Design review of the part built by this model. Coordinates are the model's own, in mm. Give positions to 0.01 mm unless a question says otherwise; leave off trailing zeros. Order: outer loops, then holes, each group sorted by start corner. A loop starts at its lowest first (then second) coordinate and runs counter-clockwise, first axis right, second up. Notation, with made-up numbers: (42.25, -33) -> (85.25, -33) arc R23 ccw to (85.25, -21) -> close; hole circle Ø2 at (64.25, 15). An arc over 180 degrees is marked (long way). One line per item, written item: value. Start each with the question number.
1) For pin 1 (0.7 mm diameter, centred on y = 3, z = 0, fed in from +X); pin 2 (0.6 mm diameter, centred on y = -2.5, z = 1, fed in from -X); pin 3 (0.7 mm diameter, centred on y = -3, z = 0, fed in from -X), all flat-tipped, find the tip position at first contact; note any pin that passes through.
2) The part is to be moulded in two halves that separate along X. For faces 1 (the face through (0.78, 0, -0.02)), 2 (the face through (-1, -1, 1.27)), 3 (the face through (2, -2.05, 0)), 4 (the face through (-2.54, -1, 0)), say which applies: released by +X, released by -X, zero draft, split by the parting line, or undercut.
3) Consider section D-D (y = -1.5). State the section outline as (x, z) points.
4) Consider section C-C (x = -1.75). State the section outline as (y, z) points, plus the area to 3 significant figures.
5) Wall thickness on line 1 along X through (y, z) = (4.75, 0.05); line 2 along Z through (x, y) = (-1.27, -4.4) (3 decimals): over which ranges is each line inside the solid? List them lowest first. Write a range as from..to.
6) Consider section A-A (y = -2.75). State the section outline as (x, z) points.
7) Consider section B-B (z = -0.55). State the section outline as (x, y) points.
from build123d import *

# Parameters (mm, degrees)
SKETCH1_W                = 0.64
SKETCH1_H                = 0.64
BOSS_EXTRUDE1_DEPTH      = 2.05
CUT_EXTRUDE1_DEPTH       = 5
SKETCH3_W                = 1.54
SKETCH3_H                = 0.5
BOSS_EXTRUDE2_DEPTH      = 0.5
SKETCH4_W                = 0.64
SKETCH4_H                = 0.64
BOSS_EXTRUDE3_DEPTH      = 5
BOSS_EXTRUDE3_DEPTH_BACK = 5.05
CHAMFER1_SIZE            = 0.2
CHAMFER1_SIZE2           = 0.115470054
CHAMFER1_PART_2_SIZE     = 0.2
CHAMFER1_PART_2_SIZE2    = 0.115470054
CHAMFER1_PART_3_SIZE     = 0.2
CHAMFER1_PART_3_SIZE2    = 0.115470054
CHAMFER1_PART_4_SIZE     = 0.2
CHAMFER1_PART_4_SIZE2    = 0.115470054
CHAMFER1_PART_5_SIZE     = 0.2
CHAMFER1_PART_5_SIZE2    = 0.115470054
CHAMFER1_PART_6_SIZE     = 0.2
CHAMFER1_PART_6_SIZE2    = 0.115470054
CHAMFER1_PART_7_SIZE     = 0.2
CHAMFER1_PART_7_SIZE2    = 0.115470054
CHAMFER1_PART_8_SIZE     = 0.2
CHAMFER1_PART_8_SIZE2    = 0.115470054
CHAMFER1_PART_9_SIZE     = 0.2
CHAMFER1_PART_9_SIZE2    = 0.115470054
CHAMFER1_PART_10_SIZE    = 0.2
CHAMFER1_PART_10_SIZE2   = 0.115470054
CHAMFER1_PART_11_SIZE    = 0.2
CHAMFER1_PART_11_SIZE2   = 0.115470054
CHAMFER1_PART_12_SIZE    = 0.2
CHAMFER1_PART_12_SIZE2   = 0.115470054
CHAMFER1_PART_13_SIZE    = 0.2
CHAMFER1_PART_13_SIZE2   = 0.115470054
CHAMFER1_PART_14_SIZE    = 0.2
CHAMFER1_PART_14_SIZE2   = 0.115470054
CHAMFER1_PART_15_SIZE    = 0.2
CHAMFER1_PART_15_SIZE2   = 0.115470054
CHAMFER1_PART_16_SIZE    = 0.2
CHAMFER1_PART_16_SIZE2   = 0.115470054
SKETCH5_R                = 0.125
CUT_EXTRUDE2_DEPTH       = 1


with BuildPart() as part:
    # Sketch1 → Boss-Extrude1 (new body)
    with BuildSketch(Plane(origin=(0, 0, 0), x_dir=(1, 0, 0), z_dir=(0, 1, 0))):
        Polygon((-2.04, -1.27), (-0.5, -1.27), (0, -0.77), (0.5, -1.27), (2.04, -1.27), (2.54, -0.77), (2.54, 0.77), (2.04, 1.27), (0.5, 1.27), (0, 0.77), (-0.5, 1.27), (-2.04, 1.27), (-2.54, 0.77), (-2.54, -0.77), align=None)
        with Locations((1.27, 0)):
            Rectangle(SKETCH1_W, SKETCH1_H, mode=Mode.SUBTRACT)
        with Locations((-1.27, 0)):
            Rectangle(SKETCH1_W, SKETCH1_H, mode=Mode.SUBTRACT)
    extrude(amount=-BOSS_EXTRUDE1_DEPTH)

    # Sketch2 → Cut-Extrude1 (cut, symmetric)
    with BuildSketch(Plane.XY):
        Polygon((-2.54, -0.2), (-2.54, 0), (-2.34, 0), align=None)
        Polygon((-0.2, 0), (0.2, 0), (0, -0.2), align=None)
        Polygon((2.34, 0), (2.54, 0), (2.54, -0.2), align=None)
        Polygon((-2.54, -1.85), (-2.34, -2.05), (-2.54, -2.05), align=None)
        Polygon((-0.2, -2.05), (0, -1.85), (0.2, -2.05), align=None)
        Polygon((2.34, -2.05), (2.54, -1.85), (2.54, -2.05), align=None)
    extrude(amount=CUT_EXTRUDE1_DEPTH, both=True, mode=Mode.SUBTRACT)

    # Sketch3 → Boss-Extrude2 (add)
    with BuildSketch(Plane.XZ.offset(2.05)):
        with Locations((-1.27, -1.02)):
            Rectangle(SKETCH3_W, SKETCH3_H)
        with Locations((-1.27, 1.02)):
            Rectangle(SKETCH3_W, SKETCH3_H)
        with Locations((1.27, 1.02)):
            Rectangle(SKETCH3_W, SKETCH3_H)
        with Locations((1.27, -1.02)):
            Rectangle(SKETCH3_W, SKETCH3_H)
    extrude(amount=BOSS_EXTRUDE2_DEPTH)

    # Sketch4 → Boss-Extrude3 (add, two sides)
    with BuildSketch(Plane(origin=(0, 0, 0), x_dir=(1, 0, 0), z_dir=(0, 1, 0))) as boss_extrude3_sk:
        with Locations((-1.27, 0)):
            Rectangle(SKETCH4_W, SKETCH4_H)
        with Locations((1.27, 0)):
            Rectangle(SKETCH4_W, SKETCH4_H)
    extrude(amount=BOSS_EXTRUDE3_DEPTH)
    extrude(boss_extrude3_sk.sketch, amount=-BOSS_EXTRUDE3_DEPTH_BACK)

    # Chamfer1
    chamfer1_edges = [part.edges().sort_by_distance(p)[0] for p in [
        (-1.59, -5.05, 0),
    ]]
    chamfer1_side = [part.faces().sort_by_distance(p)[0] for p in [
        (-1.59, -3.55, 0),
    ]]
    chamfer(chamfer1_edges, length=CHAMFER1_SIZE, length2=CHAMFER1_SIZE2, reference=chamfer1_side[0])

    # Chamfer1 part 2
    chamfer1_part_2_edges = [part.edges().sort_by_distance(p)[0] for p in [
        (-1.27, -5.05, -0.32),
    ]]
    chamfer1_part_2_side = [part.faces().sort_by_distance(p)[0] for p in [
        (-1.27, -3.55, -0.32),
    ]]
    chamfer(chamfer1_part_2_edges, length=CHAMFER1_PART_2_SIZE, length2=CHAMFER1_PART_2_SIZE2, reference=chamfer1_part_2_side[0])

    # Chamfer1 part 3
    chamfer1_part_3_edges = [part.edges().sort_by_distance(p)[0] for p in [
        (-0.95, -5.05, 0),
    ]]
    chamfer1_part_3_side = [part.faces().sort_by_distance(p)[0] for p in [
        (-0.95, -3.55, 0),
    ]]
    chamfer(chamfer1_part_3_edges, length=CHAMFER1_PART_3_SIZE, length2=CHAMFER1_PART_3_SIZE2, reference=chamfer1_part_3_side[0])

    # Chamfer1 part 4
    chamfer1_part_4_edges = [part.edges().sort_by_distance(p)[0] for p in [
        (-1.27, -5.05, 0.32),
    ]]
    chamfer1_part_4_side = [part.faces().sort_by_distance(p)[0] for p in [
        (-1.27, -3.55, 0.32),
    ]]
    chamfer(chamfer1_part_4_edges, length=CHAMFER1_PART_4_SIZE, length2=CHAMFER1_PART_4_SIZE2, reference=chamfer1_part_4_side[0])

    # Chamfer1 part 5
    chamfer1_part_5_edges = [part.edges().sort_by_distance(p)[0] for p in [
        (-1.59, 5, 0),
    ]]
    chamfer1_part_5_side = [part.faces().sort_by_distance(p)[0] for p in [
        (-1.59, 2.5, 0),
    ]]
    chamfer(chamfer1_part_5_edges, length=CHAMFER1_PART_5_SIZE, length2=CHAMFER1_PART_5_SIZE2, reference=chamfer1_part_5_side[0])

    # Chamfer1 part 6
    chamfer1_part_6_edges = [part.edges().sort_by_distance(p)[0] for p in [
        (-1.27, 5, 0.32),
    ]]
    chamfer1_part_6_side = [part.faces().sort_by_distance(p)[0] for p in [
        (-1.27, 2.5, 0.32),
    ]]
    chamfer(chamfer1_part_6_edges, length=CHAMFER1_PART_6_SIZE, length2=CHAMFER1_PART_6_SIZE2, reference=chamfer1_part_6_side[0])

    # Chamfer1 part 7
    chamfer1_part_7_edges = [part.edges().sort_by_distance(p)[0] for p in [
        (-0.95, 5, 0),
    ]]
    chamfer1_part_7_side = [part.faces().sort_by_distance(p)[0] for p in [
        (-0.95, 2.5, 0),
    ]]
    chamfer(chamfer1_part_7_edges, length=CHAMFER1_PART_7_SIZE, length2=CHAMFER1_PART_7_SIZE2, reference=chamfer1_part_7_side[0])

    # Chamfer1 part 8
    chamfer1_part_8_edges = [part.edges().sort_by_distance(p)[0] for p in [
        (-1.27, 5, -0.32),
    ]]
    chamfer1_part_8_side = [part.faces().sort_by_distance(p)[0] for p in [
        (-1.27, 2.5, -0.32),
    ]]
    chamfer(chamfer1_part_8_edges, length=CHAMFER1_PART_8_SIZE, length2=CHAMFER1_PART_8_SIZE2, reference=chamfer1_part_8_side[0])

    # Chamfer1 part 9
    chamfer1_part_9_edges = [part.edges().sort_by_distance(p)[0] for p in [
        (0.95, -5.05, 0),
    ]]
    chamfer1_part_9_side = [part.faces().sort_by_distance(p)[0] for p in [
        (0.95, -3.55, 0),
    ]]
    chamfer(chamfer1_part_9_edges, length=CHAMFER1_PART_9_SIZE, length2=CHAMFER1_PART_9_SIZE2, reference=chamfer1_part_9_side[0])

    # Chamfer1 part 10
    chamfer1_part_10_edges = [part.edges().sort_by_distance(p)[0] for p in [
        (1.27, -5.05, -0.32),
    ]]
    chamfer1_part_10_side = [part.faces().sort_by_distance(p)[0] for p in [
        (1.27, -3.55, -0.32),
    ]]
    chamfer(chamfer1_part_10_edges, length=CHAMFER1_PART_10_SIZE, length2=CHAMFER1_PART_10_SIZE2, reference=chamfer1_part_10_side[0])

    # Chamfer1 part 11
    chamfer1_part_11_edges = [part.edges().sort_by_distance(p)[0] for p in [
        (1.59, -5.05, 0),
    ]]
    chamfer1_part_11_side = [part.faces().sort_by_distance(p)[0] for p in [
        (1.59, -3.55, 0),
    ]]
    chamfer(chamfer1_part_11_edges, length=CHAMFER1_PART_11_SIZE, length2=CHAMFER1_PART_11_SIZE2, reference=chamfer1_part_11_side[0])

    # Chamfer1 part 12
    chamfer1_part_12_edges = [part.edges().sort_by_distance(p)[0] for p in [
        (1.27, -5.05, 0.32),
    ]]
    chamfer1_part_12_side = [part.faces().sort_by_distance(p)[0] for p in [
        (1.27, -3.55, 0.32),
    ]]
    chamfer(chamfer1_part_12_edges, length=CHAMFER1_PART_12_SIZE, length2=CHAMFER1_PART_12_SIZE2, reference=chamfer1_part_12_side[0])

    # Chamfer1 part 13
    chamfer1_part_13_edges = [part.edges().sort_by_distance(p)[0] for p in [
        (0.95, 5, 0),
    ]]
    chamfer1_part_13_side = [part.faces().sort_by_distance(p)[0] for p in [
        (0.95, 2.5, 0),
    ]]
    chamfer(chamfer1_part_13_edges, length=CHAMFER1_PART_13_SIZE, length2=CHAMFER1_PART_13_SIZE2, reference=chamfer1_part_13_side[0])

    # Chamfer1 part 14
    chamfer1_part_14_edges = [part.edges().sort_by_distance(p)[0] for p in [
        (1.27, 5, 0.32),
    ]]
    chamfer1_part_14_side = [part.faces().sort_by_distance(p)[0] for p in [
        (1.27, 2.5, 0.32),
    ]]
    chamfer(chamfer1_part_14_edges, length=CHAMFER1_PART_14_SIZE, length2=CHAMFER1_PART_14_SIZE2, reference=chamfer1_part_14_side[0])

    # Chamfer1 part 15
    chamfer1_part_15_edges = [part.edges().sort_by_distance(p)[0] for p in [
        (1.59, 5, 0),
    ]]
    chamfer1_part_15_side = [part.faces().sort_by_distance(p)[0] for p in [
        (1.59, 2.5, 0),
    ]]
    chamfer(chamfer1_part_15_edges, length=CHAMFER1_PART_15_SIZE, length2=CHAMFER1_PART_15_SIZE2, reference=chamfer1_part_15_side[0])

    # Chamfer1 part 16
    chamfer1_part_16_edges = [part.edges().sort_by_distance(p)[0] for p in [
        (1.27, 5, -0.32),
    ]]
    chamfer1_part_16_side = [part.faces().sort_by_distance(p)[0] for p in [
        (1.27, 2.5, -0.32),
    ]]
    chamfer(chamfer1_part_16_edges, length=CHAMFER1_PART_16_SIZE, length2=CHAMFER1_PART_16_SIZE2, reference=chamfer1_part_16_side[0])

    # Sketch5 → Cut-Extrude2 (cut)
    with BuildSketch(Plane.XZ.offset(5.05)):
        with Locations((-1.27, 0)):
            Circle(SKETCH5_R)
    extrude(amount=-CUT_EXTRUDE2_DEPTH, mode=Mode.SUBTRACT)


solid = part.part
Checked values:
1. pin 1: stops at x = 1.59
1. pin 2: stops at x = -2.04
1. pin 3: stops at x = -1.59
2. face 1: undercut
2. face 2: zero draft
2. face 3: undercut
2. face 4: released by -X
3. outline: (-2.54, -0.77) -> (-2.04, -1.27) -> (-0.5, -1.27) -> (0, -0.77) -> (0.5, -1.27) -> (2.04, -1.27) -> (2.54, -0.77) -> (2.54, 0.77) -> (2.04, 1.27) -> (0.5, 1.27) -> (0, 0.77) -> (-0.5, 1.27) -> (-2.04, 1.27) -> (-2.54, 0.77) -> close
4. outline: (-2.55, -1.27) -> (0, -1.27) -> (0, 1.27) -> (-2.55, 1.27) -> (-2.55, 0.77) -> (-2.05, 0.77) -> (-2.05, -0.77) -> (-2.55, -0.77) -> close
4. area: 5.71 mm^2
5. line 1: x = -1.59..-0.95, 0.95..1.59
5. line 2: z = -0.32..-0.125, 0.125..0.32
6. outline: (-1.59, -0.32) -> (-0.95, -0.32) -> (-0.95, 0.32) -> (-1.59, 0.32) -> close; (0.95, -0.32) -> (1.59, -0.32) -> (1.59, 0.32) -> (0.95, 0.32) -> close
7. outline: (-2.54, -1.85) -> (-2.34, -2.05) -> (-0.2, -2.05) -> (0, -1.85) -> (0.2, -2.05) -> (2.34, -2.05) -> (2.54, -1.85) -> (2.54, -0.2) -> (2.34, 0) -> (0.2, 0) -> (0, -0.2) -> (-0.2, 0) -> (-2.34, 0) -> (-2.54, -0.2) -> close
